Geometry check sheet. Reference: the model listing, model coordinates, mm. Face numbers are marked on the shaded views. A direction names the side the tool comes from. Give positions to 0.01 mm unless a question says otherwise; leave off trailing zeros. Loops run counter-clockwise (first coordinate to the right, second up) from the corner with the lowest first, then second, coordinate; pieces in that order, holes last.
1. Material ranges on L1, parallel to Z at x = 1.9, y = 0; L2, parallel to Y at x = 3.25, z = 0; L3, parallel to Z at x = 2.2, y = 14, recorded low to high.
2. Cross-section at D-D, the plane z = -4. Record the cut outline in (x, y), plus the area to 3 significant figures.
3. Tool access check on the marked faces 1, 2 and 3. Record the directions out of +Z, -Z, +X, -X, +Y, -Y that give a thin tool (end or side, any length) a straight path to the whole face; none if there is none.
4. Release check for a two-part mould opening along Z. For the marked faces 4, 5, 6 and 7 record: +Z half, -Z half, draft (parallel to the pull), parting line (faces both ways), or undercut.
5. Go/stop test with flat-tipped pins: pin 1 Ø3 at (x, y) = (2, 7.5) entering from -Z; pin 2 Ø2.5 at (x, z) = (3, 0.5) entering from -Y; pin 3 Ø1.5 at (x, z) = (3.5, 4.5) entering from +Y. Record where each tip stops, or that it passes through.
6. Cross-section at A-A, the plane z = 0. Record the cut outline in (x, y).
7. Cross-section at C-C, the plane y = 14. Record the cut outline in (x, z).
8. Cross-section at B-B, the plane y = 0. Record the cut outline in (x, z).
from build123d import *

# Parameters (mm, degrees)
BASPROSKE_W        = 5
BASPROSKE_H        = 16.5
TOOTHCUT_DEPTH     = 24.864199128
TEETHCUTS_COUNT    = 20
TEETHCUTS_ANGLE    = 342
BORSKE_R           = 2
BORE_DEPTH         = 50.0000508
CUT_EXTRUDE1_DEPTH = 10


with BuildPart() as part:
    # BasProSke → Base-Revolve (revolve)
    with BuildSketch(Plane(origin=(0, 0, 0), x_dir=(1, 0, 0), z_dir=(0, 1, 0)), mode=Mode.PRIVATE) as base_revolve_sk:
        with Locations((2.5, 8.25)):
            Rectangle(BASPROSKE_W, BASPROSKE_H)
    revolve(base_revolve_sk.sketch.rotate(Axis((-10, 0, 0), (1, 0, 0)), 180), axis=Axis((-10, 0, 0), (1, 0, 0)))

    # TooCutSke → ToothCut (cut, through all)
    with BuildSketch(Plane(origin=(0, 0, 0), x_dir=(0, 0, -1), z_dir=(1, 0, 0))):
        with BuildLine():
            ThreePointArc((0.74381438, 13.102904875), (0, 13.124), (-0.74381438, 13.102904875))
            ThreePointArc((-0.74381438, 13.102904875), (-1.226473103, 14.852072512), (-2.209965745, 16.376962373))
            ThreePointArc((-2.209965745, 16.376962373), (0, 16.5254), (2.209965745, 16.376962373))
            ThreePointArc((2.209965745, 16.376962373), (1.226473103, 14.852072512), (0.74381438, 13.102904875))
        make_face()
    toothcut = extrude(amount=TOOTHCUT_DEPTH, mode=Mode.SUBTRACT)

    # TeethCuts: ToothCut ×20 about axis
    teethcuts_axis = Axis((-10, 0, 0), (1, 0, 0))
    for i in range(1, TEETHCUTS_COUNT):
        add(toothcut.rotate(teethcuts_axis, i * TEETHCUTS_ANGLE / (TEETHCUTS_COUNT - 1)), mode=Mode.SUBTRACT)

    # BorSke → Bore (cut, symmetric)
    with BuildSketch(Plane(origin=(0, 0, 0), x_dir=(0, 0, -1), z_dir=(1, 0, 0))):
        with Locations(Location((0, 0, 0), (0, 0, 180))):
            Circle(BORSKE_R)
    extrude(amount=BORE_DEPTH, both=True, mode=Mode.SUBTRACT)

    # Sketch1 → Cut-Extrude1 (cut)
    with BuildSketch(Plane(origin=(5, 0, 0), x_dir=(0, 0, -1), z_dir=(1, 0, 0))):
        with BuildLine():
            Line((-1.428285686, 1.4), (-2.5, 1.4))
            Line((-2.5, 1.4), (-2.5, 3.4))
            Line((-2.5, 3.4), (2.5, 3.4))
            Line((2.5, 3.4), (2.5, 1.4))
            Line((2.5, 1.4), (1.428285686, 1.4))
            ThreePointArc((1.428285686, 1.4), (0, 2), (-1.428285686, 1.4))
        make_face()
    extrude(amount=-CUT_EXTRUDE1_DEPTH, mode=Mode.SUBTRACT)


solid = part.part
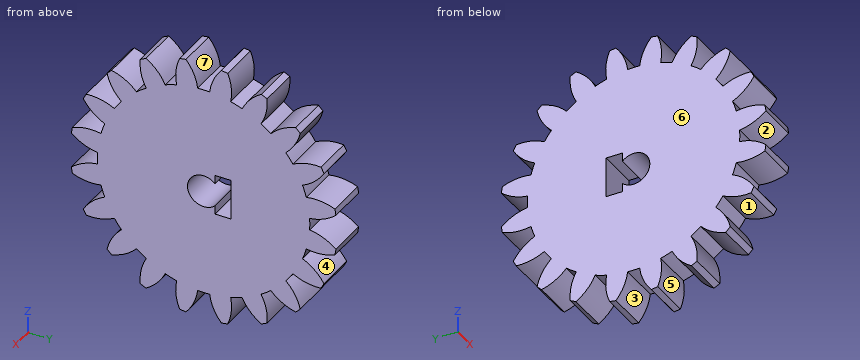
Result:
1. L1: z = -13.12 to -2, 2 to 13.12
1. L2: y = -13.12 to -2, 3.4 to 13.12
1. L3: z = -7.87 to -6, -3.46 to -0.92, 0.92 to 3.46, 6 to 7.87
2. outline: (0, -12.5) - (5, -12.5) - (5, 12.5) - (0, 12.5) - close
2. area: 125 mm2
3. face 1: +X, -X
3. face 2: +X, -X, -Y
3. face 3: -Z, +X, -X
4. face 4: undercut
4. face 5: undercut
4. face 6: draft
4. face 7: +Z half
5. pin 1: stops at z = -14.88
5. pin 2: stops at y = -15.79
5. pin 3: stops at y = 13.1
6. outline: (0, -13.12) - (5, -13.12) - (5, -2) - (0, -2) - close; (0, 3.4) - (5, 3.4) - (5, 13.12) - (0, 13.12) - close
7. outline: (0, -7.87) - (5, -7.87) - (5, -6) - (0, -6) - close; (0, -3.46) - (5, -3.46) - (5, -0.92) - (0, -0.92) - close; (0, 0.92) - (5, 0.92) - (5, 3.46) - (0, 3.46) - close; (0, 6) - (5, 6) - (5, 7.87) - (0, 7.87) - close
8. outline: (0, -13.12) - (5, -13.12) - (5, -2) - (0, -2) - close; (0, 2) - (5, 2) - (5, 13.12) - (0, 13.12) - close
